```python
from build123d import *

# Parameters (mm, degrees)
SKETCH_1_W      = 20
SKETCH_1_H      = 28
EXTRUDE_1_DEPTH = 2.7
SKETCH_2_W      = 20
SKETCH_2_H      = 28
EXTRUDE_2_DEPTH = 2.7


with BuildPart() as part:
    # 草图1 → 凸台-拉伸1 (new body)
    with BuildSketch(Plane(origin=(0, 0, 0), x_dir=(1, 0, 0), z_dir=(0, 1, 0))):
        Rectangle(SKETCH_1_W, SKETCH_1_H)
        with BuildLine():
            Line((3.25, 2), (3.25, -5))
            ThreePointArc((3.25, -5), (0, -8.25), (-3.25, -5))
            Line((-3.25, -5), (-3.25, 2))
            ThreePointArc((-3.25, 2), (0, 5.25), (3.25, 2))
        make_face(mode=Mode.SUBTRACT)
    extrude(amount=EXTRUDE_1_DEPTH)

    # 草图2 → 凸台-拉伸2 (add)
    with BuildSketch(Plane(origin=(0, 0, -14), x_dir=(-1, 0, 0), z_dir=(0, 0, -1))):
        with Locations((0, 14)):
            Rectangle(SKETCH_2_W, SKETCH_2_H)
        with BuildLine():
            Line((-3.25, 12), (-3.25, 19))
            ThreePointArc((-3.25, 19), (0, 22.25), (3.25, 19))
            Line((3.25, 19), (3.25, 12))
            ThreePointArc((3.25, 12), (0, 8.75), (-3.25, 12))
        make_face(mode=Mode.SUBTRACT)
    extrude(amount=-EXTRUDE_2_DEPTH)


solid = part.part
```
The listing builds one solid part. Answer for the finished solid, in the listing's coordinates (mm). A direction names the side the tool comes from. Round coordinates to 2 decimals unless told otherwise and drop trailing zeros. Write each loop counter-clockwise with the first axis right and the second up, starting at its lowest first coordinate (ties: lowest second). Pieces come first, ordered by that corner, then holes. Notation, with made-up numbers: (-14.75, 48) -> (32.25, 48) arc R36 cw to (32.25, 82) -> close; hole circle Ø4 at (87.25, 45). An arc over 180 degrees is marked (long way). Use CSV: the item, a comma, the result in double quotes. Start each with the question number.
(1) Section B-B on y = 10.75 is taken. Give the vertices of the cut face in (x, z), then the cut area to 3 significant figures.
(2) Section C-C on x = 0 is taken. Give the vertices of the cut face in (y, z), then the cut area to 3 significant figures.
(3) Which of the six approach directions +Z, -Z, +X, -X, +Y, -Y give full straight-line access (tool end or side, diameter ignored) to faces 4 (the face through (3.25, 1, 1)), 5 (the face through (-5, 2.7, 1)), 6 (the face through (0, 28, -13)), 7 (the face through (-5, 0, 0)), 8 (the face through (0.07, 22.25, -12.67))?
(4) Section D-D on x = -8.25 is taken. Give the vertices of the cut face in (y, z), then the cut area to 3 significant figures.
(5) Section A-A on z = 0.5 is taken. Give the vertices of the cut face in (x, y).
(6) Each of these flat-tipped pins is pushed along its axis until it touches: pin 1 (12 mm diameter, centred on x = -1.5, z = 1.5, fed in from +Y); pin 2 (4 mm diameter, centred on x = -4, y = 18.5, fed in from +Z); pin 3 (10 mm diameter, centred on x = 2, z = 9, fed in from -Y). Where does it stop, or does it pass through?
(7) The mould has two halves that part along X. Classify faces 1 (the face through (-0.07, 8.75, -12.67)), 2 (the face through (10, 2.5, -5.1)), 3 (the face through (-4, 16, -11.3)): released by +X, released by -X, zero draft, split by the parting line, or undercut.
(8) Consider L1, parallel to Y at x = -0.5, z = -9.5; L2, parallel to Z at x = 7, y = 22.25. Determine where each line is inside the solid, lowest interval first. Write a range as from..to.
A:
1,outline,"(-10, -14) -> (-3, -14) -> (-3, -11.3) -> (-10, -11.3) -> close; (3, -14) -> (10, -14) -> (10, -11.3) -> (3, -11.3) -> close"
1,area,"37.8 mm²"
2,outline,"(0, -14) -> (8.75, -14) -> (8.75, -11.3) -> (2.7, -11.3) -> (2.7, -5.25) -> (0, -5.25) -> close; (0, 8.25) -> (2.7, 8.25) -> (2.7, 14) -> (0, 14) -> close; (22.25, -14) -> (28, -14) -> (28, -11.3) -> (22.25, -11.3) -> close"
2,area,"71.0 mm²"
3,face 4,"+Y, -Y"
3,face 5,"+Z, +X, -X, +Y"
3,face 6,"+Z, -Z, +X, -X, +Y"
3,face 7,"+Z, -Z, +X, -X, -Y"
3,face 8,"+Z, -Z"
4,outline,"(0, -14) -> (28, -14) -> (28, -11.3) -> (2.7, -11.3) -> (2.7, 14) -> (0, 14) -> close"
4,area,"144 mm²"
5,outline,"(-10, 0) -> (-3.25, 0) -> (-3.25, 2.7) -> (-10, 2.7) -> close; (3.25, 0) -> (10, 0) -> (10, 2.7) -> (3.25, 2.7) -> close"
6,pin 1,"stops at y = 2.7"
6,pin 2,"stops at z = -11.3"
6,pin 3,"stops at y = 0"
7,face 1,"undercut"
7,face 2,"released by +X"
7,face 3,"zero draft"
8,L1,"y = 0..2.7"
8,L2,"z = -14..-11.3"
